```python
from build123d import *

# Parameters (mm, degrees)
SKETCH1_R           = 6.3
BASE_EXTRUDE_DEPTH  = 46
FILLET1_R           = 0.508
SHELL1_START        = 1.27
SHELL1_OUTLINE_R    = 5.03
SHELL1_DEPTH        = 43.46
SHELL1_2_OUTLINE_R  = 1.651
SHELL1_2_DEPTH      = 1.27
SKETCH3_R           = 4.78
BOSS_EXTRUDE1_DEPTH = 9.14
FILLET2_R           = 1.5
CUT_EXTRUDE1_START  = -9.14
CUT_EXTRUDE1_DEPTH  = 9.140003
FILLET6_R           = 0.254
SKETCH5_R           = 3.02
CUT_EXTRUDE2_DEPTH  = 57.108574321


# Read off the part's stored shape, not the designer's step: Shell1
with BuildPart() as part:
    # Sketch1 → Base-Extrude (new body)
    with BuildSketch(Plane.XY):
        Circle(SKETCH1_R)
    extrude(amount=BASE_EXTRUDE_DEPTH)

    # Fillet1
    fillet1_edges = [part.edges().sort_by_distance(p)[0] for p in [
        (-6.3, 0, 46),
    ]]
    fillet(fillet1_edges, radius=FILLET1_R)

    # Shell1 outline → Shell1 (cut)
    with BuildSketch(Plane.XY.offset(SHELL1_START)):
        Circle(SHELL1_OUTLINE_R)
    extrude(amount=SHELL1_DEPTH, mode=Mode.SUBTRACT)

    # Shell1 2 outline → Shell1 2 (cut)
    with BuildSketch(Plane.XY):
        Circle(SHELL1_2_OUTLINE_R)
    extrude(amount=SHELL1_2_DEPTH, mode=Mode.SUBTRACT)

    # Sketch3 → Boss-Extrude1 (add)
    with BuildSketch(Plane.XY.offset(46)):
        Circle(SKETCH3_R)
    extrude(amount=BOSS_EXTRUDE1_DEPTH)

    # Fillet2
    fillet2_edges = [part.edges().sort_by_distance(p)[0] for p in [
        (-4.78, 0, 55.14),
    ]]
    fillet(fillet2_edges, radius=FILLET2_R)

    # Sketch4 → Cut-Extrude1 (cut)
    with BuildSketch(Plane.XY.offset(55.14).offset(CUT_EXTRUDE1_START)):
        with BuildLine():
            Line((-4.364160859, 1.95), (4.364160859, 1.95))
            ThreePointArc((4.364160859, 1.95), (0, 4.78), (-4.364160859, 1.95))
        make_face()
        with BuildLine():
            Line((-4.364160859, -1.95), (4.364160859, -1.95))
            ThreePointArc((4.364160859, -1.95), (0, -4.78), (-4.364160859, -1.95))
        make_face()
    extrude(amount=CUT_EXTRUDE1_DEPTH, mode=Mode.SUBTRACT)

    # Fillet6
    fillet6_edges = [part.edges().sort_by_distance(p)[0] for p in [
        (-4.78, 0, 46),
        (0, 1.95, 46),
        (4.78, 0, 46),
        (0, -1.95, 46),
    ]]
    fillet(fillet6_edges, radius=FILLET6_R)

    # Sketch5 → Cut-Extrude2 (cut, through all)
    with BuildSketch(Plane.XZ.offset(1.95)):
        with Locations(Location((0, 50.663381062, 0), (0, 0, 270))):
            Circle(SKETCH5_R)
    extrude(amount=-CUT_EXTRUDE2_DEPTH, mode=Mode.SUBTRACT)


solid = part.part
```
Check sheet for the modelled part. Datum: model origin and axes. Units: mm. A direction names the side the tool comes from. Coordinates: 2 decimals unless noted, no trailing zeros. Loops run counter-clockwise (first coordinate to the right, second up) from the corner with the lowest first, then second, coordinate; pieces in that order, holes last. Notation, with made-up numbers: M 89.25,67.5 L 130.25,67.5 A28 ccw 130.25,92.5 Z; hole C 82,16.5 d9. An arc over 180 degrees is marked long. Answer as a JSON object with one key per item and string values.
1. Depth check by flat-ended pin: P1, Ø1.5, axis at y = 2.5, z = 33.5, coming from the -X side; P2, Ø3, axis at x = 2, y = 4, coming from the +Z side; P3, Ø7, axis at x = 0, z = 50.66, coming from the -Y side. Enter the tip coordinate at first touch or a pass-through.
Outcome:
{"P1": "x = -6.05", "P2": "z = 46", "P3": "y = -1.95"}
2. Access from +Z, -Z, +X, -X, +Y, -Y to the whole of each face (thin tool, end or side, straight path). Record for faces 1 (the cylindrical face through (-4.78, 0.03, 49.9)), 2 (the cylindrical face through (1.525, -0.632, 0.626)), 3 (the cylindrical face through (-0.655, 4.987, 22.696)), 4 (the flat face through (-3, 1.95, 49.6)), 5 (the flat face through (-3, -1.95, 49.6)).
Outcome:
{"face 1": "+Z, -X", "face 2": "-Z", "face 3": "none", "face 4": "+Z, +X, -X, +Y", "face 5": "+Z, +X, -X, -Y"}
3. Sectioned sample at C-C on z = 10.5. Record the cut outline in (x, y).
Outcome:
{"outline": "C 0,0 d12.6; hole C 0,0 d10.06"}
4. Scan lines: L1, parallel to Y at x = 0, z = 0.8; L2, parallel to Z at x = 0.25, y = 4.5; L3, parallel to X at y = 2.5, z = 28.5. Record each from-to range of solid material in increasing order. Write a range as from..to.
Outcome:
{"L1": "-6.3..-1.65, 1.65..6.3", "L2": "0..1.27, 44.73..46", "L3": "-5.78..-4.36, 4.36..5.78"}
5. Release check for a two-part mould opening along X. For faces 6 (the flat face through (1.3, -1.3, 0)), 7 (the cylindrical face through (2.546, -0.027, 49.04)), 8 (the cylindrical face through (-5, -3.83, 22.43)) record: pulls with the +X half, pulls with the -X half, needs draft (parallel to the pull), parting line crosses it, or undercut.
Outcome:
{"face 6": "needs draft", "face 7": "undercut", "face 8": "parting line crosses it"}
6. Sectioned sample at B-B on y = 0. Record the cut outline in (x, z), and give its area (3 significant figures).
Outcome:
{"outline": "M -6.3,0 L -1.65,0 L -1.65,1.27 L -5.03,1.27 L -5.03,44.73 L 5.03,44.73 L 5.03,1.27 L 1.65,1.27 L 1.65,0 L 6.3,0 L 6.3,45.49 A0.51 ccw 5.79,46 L 5.03,46 A0.25 cw 4.78,46.25 L 4.78,53.64 A1.5 ccw 3.28,55.14 L -3.28,55.14 A1.5 ccw -4.78,53.64 L -4.78,46.25 A0.25 cw -5.03,46 L -5.79,46 A0.51 ccw -6.3,45.49 Z; hole C 0,50.66 d6.04", "area": "196 mm²"}
7. Sectioned sample at A-A on x = 0. Record the cut outline in (y, z).
Outcome:
{"outline": "M -6.3,0 L -1.65,0 L -1.65,1.27 L -5.03,1.27 L -5.03,44.73 L 5.03,44.73 L 5.03,1.27 L 1.65,1.27 L 1.65,0 L 6.3,0 L 6.3,45.49 A0.51 ccw 5.79,46 L 2.2,46 A0.25 cw 1.95,46.25 L 1.95,47.64 L -1.95,47.64 L -1.95,46.25 A0.25 cw -2.2,46 L -5.79,46 A0.51 ccw -6.3,45.49 Z; M -1.95,53.68 L 1.95,53.68 L 1.95,55.14 L -1.95,55.14 Z"}
